Here's the drawing with two shaded views (mm, measured from the low corner). I have some questions. Round coordinates to 2 decimals unless told otherwise and drop trailing zeros. Write each loop counter-clockwise with the first axis right and the second up, starting at its lowest first coordinate (ties: lowest second). Pieces come first, ordered by that corner, then holes. Notation, with made-up numbers: M 86,28.25 L 131,28.25 A18 cw 131,33.25 Z; hole C 14.5,28 d4. An arc over 180 degrees is marked long. Use one line per item in the form item = value. Start each with the question number.
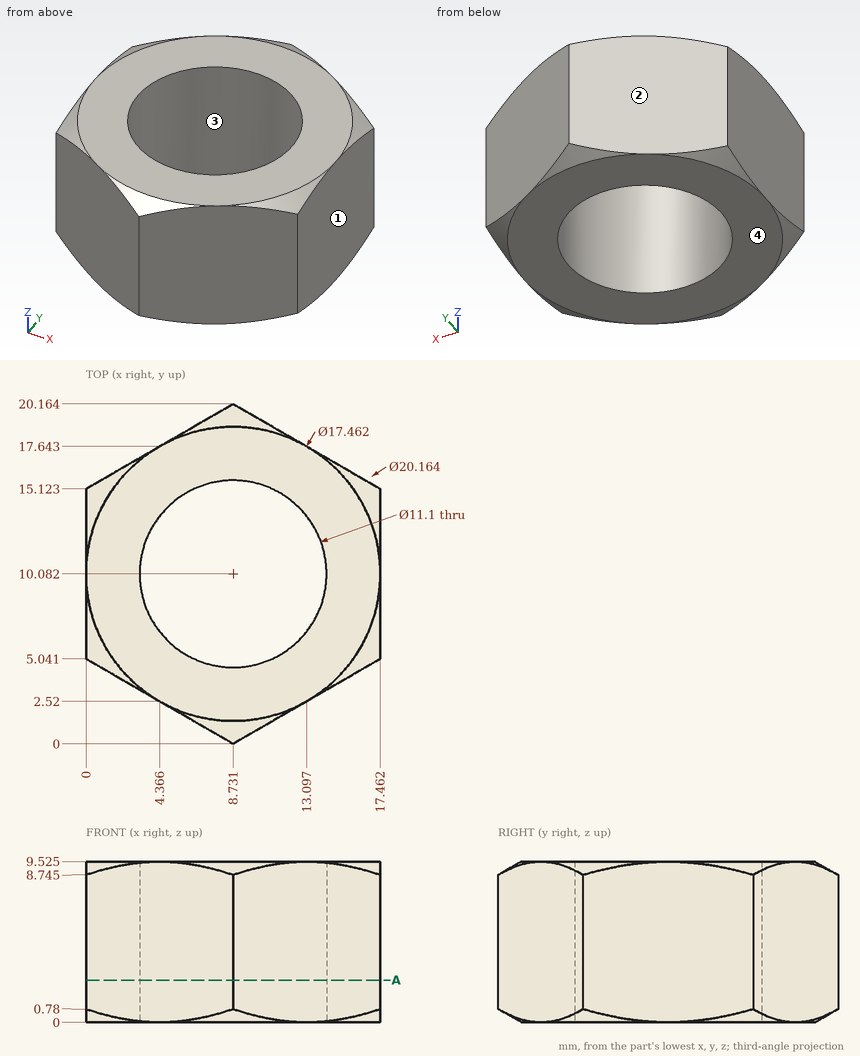
1. Will these pins go through, and if not, where does the flat tip stop? pin 1 (3 mm diameter, centred on x = 3.5, z = 2, fed in from +Y); pin 2 (5 mm diameter, centred on x = 13.5, z = 8, fed in from +Y) (1 decimal); pin 3 (1.5 mm diameter, centred on x = 2.5, z = 5.5, fed in from -Y) (1 decimal).
2. Please list where these lines run through material, in increasing order: line 1 along X through (y, z) = (13.5, 6.5) (1 decimal); line 2 along Y through (x, z) = (12.5, 7.5) (1 decimal); line 3 along Y through (x, z) = (5.5, 7.5) (1 decimal).
3. If we section it at A-A (z = 2.5): List the corners of the cut face in (x, y) for me.
4. If we mould it in two halves opening along X, with no side actions, what happens to the marked faces 1, 2, 3 and 4? For each: pulls with the +X half, pulls with the -X half, needs draft (parallel to the pull), parting line crosses it, or undercut.
Model answer:
q1.pin_1 = 18.01
q1.pin_2 = 18.9
q1.pin_3 = 3.2
q2.line_1 = 0 to 4.4, 13.1 to 17.5
q2.line_2 = 2.2 to 6, 14.2 to 18
q2.line_3 = 1.9 to 5.6, 14.6 to 18.3
q3.outline = M 0,5.04 L 8.73,0 L 17.46,5.04 L 17.46,15.12 L 8.73,20.16 L 0,15.12 Z; hole C 8.73,10.08 d11.1
q4.face_1 = pulls with the +X half
q4.face_2 = pulls with the -X half
q4.face_3 = undercut
q4.face_4 = needs draft
